Read the model definition and answer for the solid it produces. Units are mm, in the model's axes. A direction names the side the tool comes from. Round coordinates to 2 decimals unless told otherwise and drop trailing zeros. Order: outer loops, then holes, each group sorted by start corner. A loop starts at its lowest first (then second) coordinate and runs counter-clockwise, first axis right, second up. Notation, with made-up numbers: (-22.5, 80.5) - (18.5, 80.5) arc R10 cw to (18.5, 91.5) - close; hole circle Ø6 at (55, 32.25). An arc over 180 degrees is marked (long way). Answer as a JSON object with one key per item and string values. Group by question number.
Q1. A tool of negligible diameter and unlimited length cuts with its end or side. For faces 1 (the flat face through (-66.565, 2, -54)), 2 (the flat face through (-9.128, 2, -64)), 3 (the flat face through (-66.565, 2, -70)), 4 (the flat face through (-11, 2, 7.135)), from which of +Z, -Z, +X, -X, +Y, -Y can it reach the whole face along a straight path? Write none if from no direction.
Q2. A cutting plane is placed at B-B on y = 2.7. Determine the outline of the cut face in (x, z), and give its area (3 significant figures).
Q3. A cutting plane is placed at C-C on z = -52. Determine the outline of the cut face in (x, y), and give its area (3 significant figures).
Q4. Consider line 1 (Z direction, x = -69, y = 2.75); line 2 (X direction, y = 1.8, z = 0.5); line 3 (X direction, y = 2.35, z = -67). Determine where each line is inside the solid, lowest interval first.
Q5. Given pin 1 Ø1 at (y, z) = (2.5, -64) entering from +X; pin 2 Ø0.9 at (y, z) = (2, 8.5) entering from -X; pin 3 Ø1 at (y, z) = (1, 8) entering from +X, each flat-ended and moving along its own axis, determine where each tip first touches the part or whether it passes through.
Q6. The mould has two halves that part along X. Classify faces 5 (the cylindrical face through (-54.251, 1.774, -11.214)), 6 (the flat face through (-69, 2, -62.387)), 7 (the flat face through (-56.64, 1, 14.52)): pulls with the +X half, pulls with the -X half, needs draft (parallel to the pull), parting line crosses it, or undercut.
Q7. A cutting plane is placed at A-A on x = -26. Determine the outline of the cut face in (y, z).
Q8. A cutting plane is placed at D-D on x = -44.5. Determine the outline of the cut face in (y, z).
Autodesk Inventor part; units mm, degrees
ref_plane "YZ Plane" through (0, 0, 0) normal (1, 0, 0) x (0, 1, 0)
ref_plane "XZ Plane" through (0, 0, 0) normal (0, 1, 0) x (-1, 0, 0)
ref_plane "XY Plane" through (0, 0, 0) normal (0, 0, 1) x (1, 0, 0)
sketch "Sketch1" plane through (0, 0, 0) normal (0, 1, 0) x (-1, 0, 0)
  line L0 (-8.4349, 11.6133) -> (91.5651, 11.6133)
  line L1 (91.5651, 11.6133) -> (91.5651, -88.3867)
  line L2 (91.5651, -88.3867) -> (-8.4349, -88.3867)
  line L3 (-8.4349, -88.3867) -> (-8.4349, 11.6133)
  point P0 (0, 0)
  dimension "d0" = 100
  dimension "d1" = 100
extrude "Extrusion1" add sketch "Sketch1" along normal blind 3.5
sketch "Sketch2" plane through (-91.5651, 0, -88.3867) normal (-1, 0, 0) x (0, 0, 1)
  line L0 (0, 0) -> (100, 0)
  line L1 (100, 0) -> (100, 3.5)
  line L2 (0, 3.5) -> (100, 3.5)
  line L3 (0, 0) -> (0, 3.5)
  line L4 (0, 3.5) -> (100, 3.5)
  line L5 (100, 3.5) -> (90, 3.5)
  line L6 (0, 0) -> (100, 0)
  line L7 (90, 3.5) -> (100, 0)
  point P0 (88.3867, 0)
  dimension "d4" = 10
extrude "Extrusion2" cut sketch "Sketch2" against normal through all contours L7 L2 L1
sketch "Sketch3" plane through (0, 3.5, 0) normal (0, 1, 0) x (1, 0, 0)
  line L0 (-91.5651, -1.6133) -> (8.4349, -1.6133)
  line L1 (8.4349, -1.6133) -> (8.4349, 88.3867)
  line L2 (8.4349, 88.3867) -> (-91.5651, 88.3867)
  line L3 (-91.5651, 88.3867) -> (-91.5651, -1.6133)
  line L4 (8.4349, -1.6133) -> (8.4349, -11.6133)
  line L5 (-91.5651, -1.6133) -> (8.4349, -1.6133)
  line L6 (-91.5651, -11.6133) -> (-91.5651, -1.6133)
  line L7 (-91.5651, -11.6133) -> (8.4349, -11.6133)
  line L8 (-91.5651, -11.6133) -> (8.4349, -11.6133)
  line L9 (8.4349, 88.3867) -> (-91.5651, 88.3867)
  line L10 (-91.5651, 88.3867) -> (-91.5651, -11.6133)
  line L11 (-41.5651, -11.6133) -> (8.4349, -11.6133)
  line L12 (-91.5651, -11.6133) -> (-41.5651, -11.6133)
  line L13 (-16.5651, -11.6133) -> (8.4349, -11.6133)
  line L14 (-91.5651, -11.6133) -> (-66.5651, -11.6133)
  line L15 (-16.5651, -11.6133) -> (-4.0651, -11.6133)
  line L16 (-79.0651, -11.6133) -> (-66.5651, -11.6133)
  line L17 (-41.5651, 25.8867) -> (-72.8151, -11.6133)
  line L18 (-41.5651, 25.8867) -> (-10.3151, -11.6133)
  line L19 (-28.2288, 9.8831) -> (-18.6484, -1.6133)
  line L20 (-91.5651, -1.6133) -> (8.4349, -1.6133)
  circle A0 centre (-30.1493, 12.1878) radius 1.6
  circle A1 centre (-20.569, 0.6914) radius 1.6
  line L21 (-18.6484, -1.6133) -> (-20.569, 0.6914)
  line L22 (-41.5651, 25.8867) -> (-41.5651, -11.6133)
  circle A2 centre (-52.9808, 12.1878) radius 1.6
  circle A3 centre (-62.5612, 0.6914) radius 1.6
  point P0 (0, 0)
  point P1 (-63.1373, 0)
  dimension "d15" = 3.2
  dimension "d16" = 3.2
  dimension "d17" = 3
extrude "Extrusion3" cut sketch "Sketch3" against normal through all contours A1 L18 | L18 A1 | A3 L17 | L17 A3 | A2 L17 | L17 A2 | A0 L18 | L18 A0
sketch "Sketch4" plane through (0, 0, 0) normal (0, -1, 0) x (1, 0, 0)
  circle A0 centre (-52.9808, -12.1878) radius 1.6
  circle A1 centre (-20.569, -0.6914) radius 1.6
  circle A2 centre (-62.5612, -0.6914) radius 1.6
  circle A3 centre (-30.1493, -12.1878) radius 1.6
  line L0 (8.4349, -88.3867) -> (-91.5651, -88.3867)
  line L1 (8.4349, 11.6133) -> (8.4349, -88.3867)
  line L2 (-91.5651, 11.6133) -> (8.4349, 11.6133)
  line L3 (-91.5651, -88.3867) -> (-91.5651, 11.6133)
  line L4 (-91.5651, -88.3867) -> (-91.5651, 11.6133)
  line L5 (-91.5651, 11.6133) -> (8.4349, 11.6133)
  line L6 (8.4349, 11.6133) -> (8.4349, 21.6133)
  line L7 (8.4349, 21.6133) -> (-91.5651, 21.6133)
  line L8 (-91.5651, 21.6133) -> (-91.5651, 11.6133)
  line L9 (8.4349, 11.6133) -> (8.4349, -88.3867)
  line L10 (-91.5651, -88.3867) -> (8.4349, -88.3867)
  line L11 (8.4349, -88.3867) -> (8.4349, -78.3867)
  line L12 (8.4349, -78.3867) -> (-91.5651, -78.3867)
  line L13 (-91.5651, -78.3867) -> (-91.5651, -88.3867)
  line L14 (-91.5651, 1.6133) -> (8.4349, 1.6133)
  line L15 (-91.5651, 11.6133) -> (8.4349, 11.6133)
  line L16 (8.4349, 11.6133) -> (8.4349, 1.6133)
  line L17 (8.4349, 1.6133) -> (-91.5651, 1.6133)
  line L18 (-91.5651, 1.6133) -> (-91.5651, 11.6133)
  ellipse E0 centre (-76.8987, 15.9252) end of major axis (-87.6538, 6.9626) minor radius 2.0831
  point P0 (0, 0)
  dimension "d20" = 10
  dimension "d21" = 10
extrude "Extrusion4" add sketch "Sketch4" against normal up to surface (3.5 mm away) contours L14 L3 L2 E0 L1 | L2 E0 L7 L6 | L8 L7 E0 L2 | E0 L2 | L2 E0 L7
sketch "Sketch5" plane through (0, 0, 0) normal (0, -1, 0) x (1, 0, 0)
  line L0 (-91.5651, -88.3867) -> (-91.5651, 21.6133)
  line L1 (8.4349, -88.3867) -> (-91.5651, -88.3867)
  line L2 (8.4349, -88.3867) -> (8.4349, 21.6133)
  line L3 (8.4349, 21.6133) -> (-91.5651, 21.6133)
  circle A0 centre (-30.1493, -12.1878) radius 1.6
  circle A1 centre (-62.5612, -0.6914) radius 1.6
  circle A2 centre (-20.569, -0.6914) radius 1.6
  circle A3 centre (-52.9808, -12.1878) radius 1.6
  line L4 (-91.5651, -88.3867) -> (-91.5651, 21.6133)
  line L5 (8.4349, -88.3867) -> (-91.5651, -88.3867)
  line L6 (-91.5651, -88.3867) -> (-91.5651, -78.3867)
  line L7 (-91.5651, -78.3867) -> (8.4349, -78.3867)
  line L8 (8.4349, -78.3867) -> (8.4349, -88.3867)
  point P0 (0, 0)
  dimension "d24" = 10
extrude "Extrusion5" cut sketch "Sketch5" against normal through all contours L0 L7 L2 L1
sketch "Sketch6" plane through (-91.5651, 0, 21.6133) normal (-1, 0, 0) x (0, 0, 1)
  line L0 (-100, 3.5) -> (-100, 0)
  line L1 (-100, 0) -> (0, 0)
  line L2 (0, 0) -> (0, 3.5)
  line L3 (0, 3.5) -> (-100, 3.5)
  line L4 (-6.5312, 3.5) -> (-20.2018, 3.5)
  line L5 (-6.5312, 8.5) -> (-6.5312, 3.5)
  line L6 (-20.2018, 8.5) -> (-6.5312, 8.5)
  line L7 (-20.2018, 3.5) -> (-20.2018, 8.5)
  line L8 (-100, 0) -> (0, 0)
  line L9 (0, 0) -> (-11.4782, 3.5)
  line L10 (0, 3.5) -> (-100, 3.5)
  point P0 (-21.6133, 0)
  dimension "d27" = 12
extrude "Extrusion6" cut sketch "Sketch6" against normal through all contours L9 L3 L2
sketch "Sketch7" plane through (0, 3.5, 0) normal (0, 1, 0) x (1, 0, 0)
  line L0 (-91.5651, -10.1351) -> (8.4349, -10.1351)
  line L1 (8.4349, -10.1351) -> (8.4349, 78.3867)
  line L2 (8.4349, 78.3867) -> (-91.5651, 78.3867)
  line L3 (-91.5651, -10.1351) -> (-91.5651, 78.3867)
  circle A0 centre (-52.9808, 12.1878) radius 1.6
  circle A1 centre (-20.569, 0.6914) radius 1.6
  circle A2 centre (-62.5612, 0.6914) radius 1.6
  circle A3 centre (-30.1493, 12.1878) radius 1.6
  line L4 (8.4349, -10.1351) -> (8.4349, -21.6133)
  line L5 (-91.5651, -10.1351) -> (8.4349, -10.1351)
  line L6 (-91.5651, -21.6133) -> (-91.5651, -10.1351)
  line L7 (8.4349, -21.6133) -> (-91.5651, -21.6133)
  circle A4 centre (-30.1493, 12.1878) radius 1.6
  circle A5 centre (-20.569, 0.6914) radius 1.6
  line L8 (-30.1493, 12.1878) -> (-20.569, 0.6914)
  line L9 (-91.5651, -10.1351) -> (8.4349, -10.1351)
  line L10 (-30.1493, -10.1351) -> (-20.569, -21.6133)
  line L11 (8.4349, -21.6133) -> (-91.5651, -21.6133)
  circle A6 centre (-62.5612, 0.6914) radius 1.6
  line L12 (-52.9808, 12.1878) -> (-62.5612, 0.6914)
  line L13 (-52.9808, -10.1351) -> (-62.5612, -21.6133)
  point P0 (0, 0)
extrude "Extrusion7" cut sketch "Sketch7" against normal blind 10 contours L0 L13 L7 L6 | L0 L4 L7 L10
sketch "Sketch8" plane through (0, 3.5, 0) normal (0, 1, 0) x (1, 0, 0)
  line L0 (-91.5651, -10.1351) -> (-52.9808, -10.1351)
  line L1 (-52.9808, -10.1351) -> (-30.1493, -10.1351)
  line L2 (-30.1493, -10.1351) -> (8.4349, -10.1351)
  line L3 (8.4349, -10.1351) -> (8.4349, 78.3867)
  line L4 (8.4349, 78.3867) -> (-91.5651, 78.3867)
  line L5 (-91.5651, -10.1351) -> (-91.5651, 78.3867)
  circle A0 centre (-52.9808, 12.1878) radius 1.6
  circle A1 centre (-20.569, 0.6914) radius 1.6
  circle A2 centre (-62.5612, 0.6914) radius 1.6
  circle A3 centre (-30.1493, 12.1878) radius 1.6
  line L6 (8.4349, -10.1351) -> (8.4349, 78.3867)
  line L7 (8.4349, -10.1351) -> (-30.1493, -10.1351)
  line L8 (-30.1493, -10.1351) -> (-30.1493, -7.1351)
  line L9 (-30.1493, -7.1351) -> (8.4349, -7.1351)
  line L10 (8.4349, -7.1351) -> (8.4349, -10.1351)
  line L11 (-91.5651, -10.1351) -> (-52.9808, -10.1351)
  line L12 (-52.9808, -10.1351) -> (-52.9808, -7.1351)
  line L13 (-52.9808, -7.1351) -> (-91.5651, -7.1351)
  line L14 (-91.5651, -7.1351) -> (-91.5651, -10.1351)
  point P0 (0, 0)
  dimension "d32" = 3
extrude "Extrusion8" cut sketch "Sketch8" against normal through all contours L5 L13 L12 L0 | L8 L9 L3 L2
sketch "Sketch9" plane through (0, 3.5, 0) normal (0, 1, 0) x (1, 0, 0)
  circle A0 centre (-30.1493, 12.1878) radius 1.6
  circle A1 centre (-62.5612, 0.6914) radius 1.6
  circle A2 centre (-20.569, 0.6914) radius 1.6
  circle A3 centre (-52.9808, 12.1878) radius 1.6
  line L0 (-91.5651, -7.1351) -> (-52.9808, -7.1351)
  line L1 (-52.9808, -7.1351) -> (-52.9808, -10.1351)
  line L2 (-52.9808, -10.1351) -> (-30.1493, -10.1351)
  line L3 (-30.1493, -10.1351) -> (-30.1493, -7.1351)
  line L4 (-30.1493, -7.1351) -> (8.4349, -7.1351)
  line L5 (8.4349, -7.1351) -> (8.4349, 78.3867)
  line L6 (8.4349, 78.3867) -> (-91.5651, 78.3867)
  line L7 (-91.5651, -7.1351) -> (-91.5651, 78.3867)
  line L8 (-91.5651, 78.3867) -> (-91.5651, -7.1351)
  line L9 (8.4349, 78.3867) -> (8.4349, -7.1351)
  line L10 (-91.5651, 78.3867) -> (8.4349, 78.3867)
  line L11 (8.4349, 78.3867) -> (8.4349, 73.3867)
  line L12 (8.4349, 73.3867) -> (-91.5651, 73.3867)
  line L13 (-91.5651, 73.3867) -> (-91.5651, 78.3867)
  line L14 (-91.5651, 78.3867) -> (8.4349, 78.3867)
  line L15 (-41.5651, 78.3867) -> (-41.5651, 59.9995)
  line L16 (-41.5651, 59.9995) -> (-16.5651, 59.9995)
  line L17 (-16.5651, 59.9995) -> (-66.5651, 59.9995)
  line L18 (8.4349, 73.3867) -> (-16.5651, 73.3867)
  line L19 (-16.5651, 73.3867) -> (-16.5651, 45.3867)
  line L20 (-16.5651, 45.3867) -> (8.4349, 45.3867)
  line L21 (8.4349, 45.3867) -> (8.4349, 73.3867)
  line L22 (-66.5651, 73.3867) -> (-79.5403, 73.3867)
  line L23 (-79.5403, 73.3867) -> (-79.5403, 45.3867)
  line L24 (-79.5403, 45.3867) -> (-66.5651, 45.3867)
  line L25 (-66.5651, 45.3867) -> (-66.5651, 73.3867)
  line L26 (-91.5651, 45.3867) -> (-66.5651, 45.3867)
  line L27 (-66.5651, 45.3867) -> (-66.5651, 78.3867)
  line L28 (-66.5651, 78.3867) -> (-91.5651, 78.3867)
  line L29 (-91.5651, 78.3867) -> (-91.5651, 45.3867)
  line L30 (-14.4969, 45.3867) -> (-14.4969, 50.3867)
  line L31 (-14.4969, 50.3867) -> (-14.4969, 78.3867)
  line L32 (-14.4969, 64.3867) -> (-82.4701, 64.3867)
  line L33 (-82.4701, 64.3867) -> (-3.1512, 64.3867)
  line L34 (-14.4969, 64.3867) -> (-9.1279, 64.3867)
  line L35 (-9.1279, 64.3867) -> (-9.1279, 62.3867)
  line L36 (-9.1279, 62.3867) -> (-14.4969, 62.3867)
  line L37 (-14.4969, 62.3867) -> (-14.4969, 64.3867)
  line L38 (-14.4969, 64.3867) -> (-9.1279, 64.3867)
  line L39 (-9.1279, 64.3867) -> (-9.1279, 66.3867)
  line L40 (-9.1279, 66.3867) -> (-14.4969, 66.3867)
  line L41 (-14.4969, 66.3867) -> (-14.4969, 64.3867)
  line L42 (-66.5651, 64.3867) -> (-72.2729, 64.3867)
  line L43 (-72.2729, 64.3867) -> (-72.2729, 62.3867)
  line L44 (-72.2729, 62.3867) -> (-66.5651, 62.3867)
  line L45 (-66.5651, 62.3867) -> (-66.5651, 64.3867)
  line L46 (-72.2729, 62.3867) -> (-66.5651, 62.3867)
  line L47 (-66.5651, 62.3867) -> (-66.5651, 66.3867)
  line L48 (-66.5651, 66.3867) -> (-72.2729, 66.3867)
  line L49 (-72.2729, 66.3867) -> (-72.2729, 62.3867)
  line L50 (-14.4969, 73.3867) -> (-14.4969, 66.3867)
  line L51 (-9.1279, 66.3867) -> (-14.4969, 66.3867)
  line L52 (-9.1279, 66.3867) -> (-9.1279, 62.3867)
  line L53 (-14.4969, 62.3867) -> (-14.4969, 45.3867)
  line L54 (-14.4969, 62.3867) -> (-9.1279, 62.3867)
  line L55 (-14.4969, 45.3867) -> (8.4349, 45.3867)
  line L56 (-14.4969, 66.3867) -> (-16.5651, 66.3867)
  line L57 (-14.4969, 62.3867) -> (-16.5651, 62.3867)
  point P0 (0, 0)
  dimension "d35" = 5
  dimension "d36" = 25
  dimension "d37" = 50
  dimension "d38" = 28
  dimension "d39" = 28
  dimension "d40" = 5
  dimension "d41" = 2
  dimension "d42" = 2
extrude "Extrusion9" cut sketch "Sketch9" against normal through all contours L7 L12 L23 L26 | L7 L6 L27 L12 | L23 L32 L43 L44 L25 L24 | L12 L25 L48 L49 L32 L23 | L6 L15 L12 L27 | L6 L31 L12 L15 | L20 L30 L31 L36 L35 L39 L40 L12 L5 | L6 L5 L12 L31 | L12 L31 L56 L19 | L19 L57 L31 L30 L20
properties material "Steel, Alloy"
Result set:
{
 "1": {"face 1": "-X, +Y, -Y", "face 2": "-Z, +X, +Y, -Y", "face 3": "-Z, -X, +Y, -Y", "face 4": "+X, +Y, -Y"},
 "2": {"outline": "(-91.57, -45.39) - (-66.57, -45.39) - (-66.57, -62.39) - (-72.27, -62.39) - (-72.27, -66.39) - (-66.57, -66.39) - (-66.57, -73.39) - (-16.57, -73.39) - (-16.57, -66.39) - (-9.13, -66.39) - (-9.13, -62.39) - (-16.57, -62.39) - (-16.57, -45.39) - (8.43, -45.39) - (8.43, 7.14) - (-30.15, 7.14) - (-30.15, 10.14) - (-27.96, 12.76) - (-55.17, 12.76) - (-52.98, 10.14) - (-52.98, 7.14) - (-91.57, 7.14) - close; hole circle Ø3.2 at (-62.56, -0.69); hole circle Ø3.2 at (-52.98, -12.19); hole circle Ø3.2 at (-30.15, -12.19); hole circle Ø3.2 at (-20.57, -0.69)", "area": "6,810 mm²"},
 "3": {"outline": "(-66.57, 0) - (-16.57, 0) - (-16.57, 3.5) - (-66.57, 3.5) - close", "area": "175 mm²"},
 "4": {"line 1": "z = -66.39 to -62.39, -45.39 to 7.14", "line 2": "x = -91.57 to -63.63, -61.49 to -21.64, -19.5 to 8.43", "line 3": "x = -66.57 to -16.57"},
 "5": {"pin 1": "stops at x = -9.13", "pin 2": "stops at x = -52.98", "pin 3": "stops at x = -30.15"},
 "6": {"face 5": "undercut", "face 6": "needs draft", "face 7": "pulls with the -X half"},
 "7": {"outline": "(0, -73.39) - (3.5, -73.39) - (3.5, 7.14) - (0, 7.14) - close; (0, 15.11) - (1.98, 15.11) - (0, 21.61) - close"},
 "8": {"outline": "(0, -73.39) - (3.5, -73.39) - (3.5, 10.14) - (0, 21.61) - close"}
}
